Autodesk Inventor part; units mm, degrees
ref_plane "YZ Plane" through (0, 0, 0) normal (1, 0, 0) x (0, 1, 0)
ref_plane "XZ Plane" through (0, 0, 0) normal (0, 1, 0) x (-1, 0, 0)
ref_plane "XY Plane" through (0, 0, 0) normal (0, 0, 1) x (1, 0, 0)
ref_plane "Work Plane13" through (-2.54, 44.7855, -14.3129) normal (0, -1, 0) x (1, 0, 0)
sketch "Sketch6" plane through (-2.54, 44.7855, -14.3129) normal (0, -1, 0) x (1, 0, 0)
  line L0 (6.35, 32.4159) -> (26.9875, 32.4159)
  line L1 (13.4874, 32.4159) -> (13.4874, 26.0989)
  line L2 (26.9875, 32.4159) -> (26.9875, -3.9117)
  point P0 (2.54, 14.3129)
  dimension "d20" = 13.5001
ref_plane "Work Plane14" through (-2.54, 0, 0) normal (-1, 0, 0) x (0, 0, 1)
sketch "Sketch15" plane through (-2.54, 0, 0) normal (-1, 0, 0) x (0, 0, 1)
  circle A0 centre (0, 0) radius 41.275
  circle A1 centre (0, 0) radius 44.45
  dimension "d47" = 82.55
  dimension "d48" = 88.9
extrude "Extrusion11" add sketch "Sketch15" against normal blind 2.54
ref_plane "Work Plane10" through (0, 0, 0) normal (1, 0, 0) x (0, 0, -1)
sketch "Sketch16" plane through (0, 0, 0) normal (1, 0, 0) x (0, 0, -1)
  circle A0 centre (0, 0) radius 44.45
  circle A1 centre (0, 0) radius 41.275
  dimension "d51" = 82.55
extrude "Extrusion12" add sketch "Sketch16" along normal blind 31.75
ref_plane "Work Plane9" through (-2.54, 0, 0) normal (-1, 0, 0) x (0, 0, 1)
sketch "Sketch19" plane through (-2.54, 0, 0) normal (-1, 0, 0) x (0, 0, 1)
  line L0 (4.3346, 1.4542) -> (-4.3346, 1.4542)
  arc A0 (-16.671, 37.7585) -> (16.671, 37.7585) centre (0, 0) ccw
  line L1 (-4.3346, 1.4542) -> (-41.2494, 1.4542)
  line L2 (4.3346, 1.4542) -> (41.2494, 1.4542)
  circle A1 centre (0, 0) radius 8.382
  line L3 (-4.3346, -1.4542) -> (4.3346, -1.4542)
  line L4 (4.3346, 1.4542) -> (-4.3346, 1.4542)
  line L5 (-41.2494, -1.4542) -> (41.2494, -1.4542)
extrude "Extrusion14" add sketch "Sketch19" against normal blind 6.35 contours L2 A1 L5 L3 L1 L0 | L2 A0 L5 A1 | A1 L5 A0 L1
sketch "Sketch20" plane through (3.81, 0, 0) normal (1, 0, 0) x (0, 0, -1)
  line L0 (41.2494, 1.4542) -> (-41.2494, 1.4542)
  line L1 (-41.2494, -1.4542) -> (41.2494, -1.4542)
  arc A0 (-41.2494, 1.4542) -> (-41.2494, -1.4542) centre (0, 0) ccw
  arc A1 (41.2494, -1.4542) -> (41.2494, 1.4542) centre (0, 0) ccw
extrude "Extrusion15" cut sketch "Sketch20" against normal blind 6.35
ref_plane "Work Plane12" through (-2.54, 0, 0) normal (-1, 0, 0) x (0, 0, 1)
ref_plane "Work Plane11" through (3.81, 0, 0) normal (1, 0, 0) x (0, 0, -1)
properties part number "LiftMotorHousingBottom[FINAL]"
Geometry check sheet. Reference: the model listing, model coordinates, mm. A direction names the side the tool comes from. Give positions to 0.01 mm unless a question says otherwise; leave off trailing zeros. Order: outer loops, then holes, each group sorted by start corner. A loop starts at its lowest first (then second) coordinate and runs counter-clockwise, first axis right, second up.
1) Gauge pin test, flat ends, axial feed: pin 1 (8 mm diameter, centred on x = 24.5, y = 34.5, fed in from +Z) (3 decimals); pin 2 (8 mm diameter, centred on x = 20.5, y = 32.5, fed in from +Z); pin 3 (5 mm diameter, centred on x = 3.5, z = -12.5, fed in from -Y); pin 4 (10 mm diameter, centred on y = -6.5, z = -33.5, fed in from +X). Record the tip position at first contact, or that the pin passes through.
Results are:
pin 1: stops at z = 32.335
pin 2: stops at z = 34.11
pin 3: stops at y = -43.31
pin 4: passes through
2) Cross-section at B-B (y = -20). Record the boundary of the cut face in (x, z).
Results are:
outline: (-2.54, -39.7) - (31.75, -39.7) - (31.75, -36.11) - (-2.54, -36.11) - close; (-2.54, 36.11) - (31.75, 36.11) - (31.75, 39.7) - (-2.54, 39.7) - close
3) Cross-section at C-C (x = 25). Record the boundary of the cut face in (y, z) (3 decimals).
Results are:
outline: circle Ø88.9 at (0, 0); hole circle Ø82.55 at (0, 0)
4) Cross-section at A-A (z = 0). Record the boundary of the cut face in (x, y) (3 decimals), then the cut area to 3 significant figures.
Results are:
outline: (-2.54, -44.45) - (31.75, -44.45) - (31.75, -41.275) - (-2.54, -41.275) - close; (-2.54, 41.275) - (31.75, 41.275) - (31.75, 44.45) - (-2.54, 44.45) - close
area: 218 mm2
5) Draft check along Y on faces 3 (the cylindrical face through (0.679, 0.02, 41.275)), 4 (the flat face through (-2.54, -29.4, 29.4)). Enter one of: released by +Y, released by -Y, zero draft, split by the parting line, or undercut.
Results are:
face 3: undercut
face 4: zero draft
6) Material ranges on probe 1 along Y at (x, z) = (9, 0) (3 decimals); probe 2 along Y at (x, z) = (16.5, 11.5), recorded low to high.
Results are:
probe 1: y = -44.45 to -41.275, 41.275 to 44.45
probe 2: y = -42.94 to -39.64, 39.64 to 42.94
7) Tool access check on faces 1 (the flat face through (31.75, -29.4, -29.4)), 2 (the cylindrical face through (0.679, -0.02, -41.275)). Record the directions out of +Z, -Z, +X, -X, +Y, -Y that give a thin tool (end or side, any length) a straight path to the whole face; none if there is none.
Results are:
face 1: +Z, -Z, +X, +Y, -Y
face 2: +X, -X
